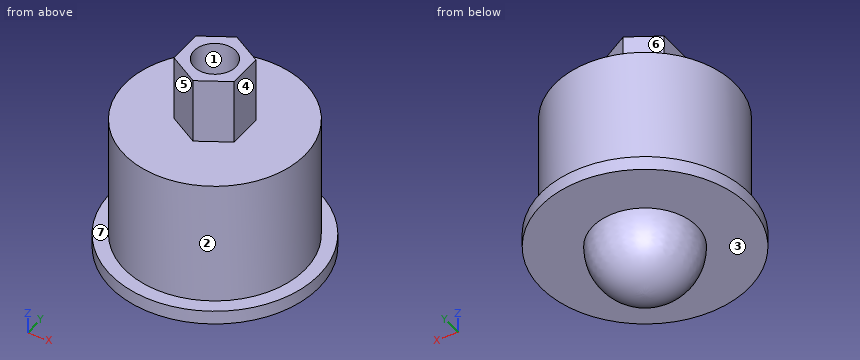
```python
from build123d import *

# Parameters (mm, degrees)
F2_R     = 1.5
F3_DEPTH = 4.75


with BuildPart() as f1:
    # F0 (on Front) → F1 (revolve)
    with BuildSketch(Plane.XZ):
        with BuildLine():
            Line((0, 0), (0, -3.75))
            ThreePointArc((0, -3.75), (2.65165, -2.65165), (3.75, 0))
            Line((3.75, 0), (0, 0))
        make_face()
        with BuildLine():
            Line((0, 0), (3.75, 0))
            ThreePointArc((3.75, 0), (2.65165, 2.65165), (0, 3.75))
            Line((0, 3.75), (0, 0))
        make_face()
        with BuildLine():
            ThreePointArc((0, 3.75), (2.65165, 2.65165), (3.75, 0))
            Line((3.75, 0), (7.5, 0))
            Line((7.5, 0), (7.5, 1))
            Line((7.5, 1), (6.5, 1))
            Line((6.5, 1), (6.5, 10))
            Line((6.5, 10), (0, 10))
            Line((0, 10), (0, 3.75))
        make_face()
    revolve(axis=Axis((0, 0, 3.125), (0, 0, -1)))

    # F2 (on face) → F3 (join)
    with BuildSketch(Plane.XY.offset(10)):
        Polygon((2.165064, 1.25), (0, 2.5), (-2.165064, 1.25), (-2.165064, -1.25), (0, -2.5), (2.165064, -1.25), align=None)
        Circle(F2_R, mode=Mode.SUBTRACT)
    extrude(amount=F3_DEPTH)


solid = f1.part
```
Verification items for the finished model (mm, model axes). Face numbers are marked on the shaded views. A direction names the side the tool comes from. Round coordinates to 2 decimals unless told otherwise and drop trailing zeros. Loops run counter-clockwise (first coordinate to the right, second up) from the corner with the lowest first, then second, coordinate; pieces in that order, holes last. Notation, with made-up numbers: (-2.5, 50) -> (1.5, 50) arc R31 cw to (1.5, 89) -> close; hole circle Ø3 at (2, 10.25). An arc over 180 degrees is marked (long way). Answer as a JSON object with one key per item and string values.
Q1. Scan lines: line 1 (Z direction, x = 0, y = 6.75); line 2 (Z direction, x = -6, y = 1.5); line 3 (X direction, y = 0.5, z = 12.25). Record each from-to range of solid material in increasing order. Write a range as from..to.
Data:
{"line 1": "z = 0..1", "line 2": "z = 0..10", "line 3": "x = -2.17..-1.41, 1.41..2.17"}
Q2. Section check A-A (y = 5). Record the boundary of the cut face in (x, z).
Data:
{"outline": "(-5.59, 0) -> (5.59, 0) -> (5.59, 1) -> (4.15, 1) -> (4.15, 10) -> (-4.15, 10) -> (-4.15, 1) -> (-5.59, 1) -> close"}
Q3. Access from +Z, -Z, +X, -X, +Y, -Y to the whole of each face (thin tool, end or side, straight path). Record for the marked faces 4, 5, 6 and 7.
Data:
{"face 4": "+Z, +X, +Y, -Y", "face 5": "+Z, -X, -Y", "face 6": "+Z, -X, +Y", "face 7": "+Z"}
Q4. Go/stop test with flat-tipped pins: P1, Ø7.5, axis at x = -2.5, y = 2, coming from the +Z side; P2, Ø1.2, axis at y = 0, z = 12.5, coming from the -X side; P3, Ø5, axis at y = -4.5, z = 8.5, coming from the -X side; P4, Ø3, axis at x = 5.5, z = 4.5, coming from the +Y side. Record where each tip stops, or that it passes through.
Data:
{"P1": "stops at z = 14.75", "P2": "stops at x = -2.17", "P3": "stops at x = -6.18", "P4": "stops at y = 5.12"}
Q5. Section check B-B (z = 9.25). Record the boundary of the cut face in (x, y).
Data:
{"outline": "circle Ø13 at (0, 0)"}
Q6. Section check C-C (y = -4). Record the boundary of the cut face in (x, z), then the cut area to 3 significant figures.
Data:
{"outline": "(-6.34, 0) -> (6.34, 0) -> (6.34, 1) -> (5.12, 1) -> (5.12, 10) -> (-5.12, 10) -> (-5.12, 1) -> (-6.34, 1) -> close", "area": "105 mm2"}
Q7. Section check D-D (z = 0.75). Record the boundary of the cut face in (x, y), then the cut area to 3 significant figures.
Data:
{"outline": "circle Ø15 at (0, 0)", "area": "177 mm2"}
Q8. Draft check along X on the marked faces 1, 2 and 3. Enter one of: pulls with the +X half, pulls with the -X half, needs draft (parallel to the pull), parting line crosses it, or undercut.
Data:
{"face 1": "undercut", "face 2": "parting line crosses it", "face 3": "needs draft"}
